Autodesk Fusion 360 part; units mm, degrees
sketch "Dimension" plane through (0, 0, 0) normal (0, 1, 0) x (1, 0, 0)
  line L0 (50, -40) -> (-50, -40)
  line L1 (-50, -40) -> (-50, 40)
  line L2 (-50, 40) -> (50, 40)
  line L3 (50, 40) -> (50, -40)
  line L4 (50, -40) -> (-50, 40) construction
  line L5 (-50, -40) -> (50, 40) construction
  dimension "d4" = 100
  dimension "d5" = 80
extrude "Extrude1" add sketch "Dimension" along normal blind 3
sketch "Stepper Mount" plane through (0, 3, 0) normal (0, 1, 0) x (-1, 0, 0)
  line L0 (-50, -40) -> (50, -40)
  line L1 (50, -40) -> (50, 40)
  line L2 (50, 40) -> (-50, 40)
  line L3 (-50, 40) -> (-50, -40)
  line L4 (30, -40) -> (-30, -40)
  line L5 (-30, -40) -> (-30, 40) construction
  line L6 (-30, 40) -> (30, 40)
  line L7 (30, 40) -> (30, -40) construction
  circle A0 centre (23.55, -33.85) radius 2.55
  circle A1 centre (-23.55, -33.85) radius 2.55
  circle A2 centre (23.55, 13.25) radius 2.55
  circle A3 centre (-23.55, 13.25) radius 2.55
  line L8 (-23.55, 13.25) -> (23.55, -33.85)
  circle A4 centre (15.49, -25.79) radius 2
  line L9 (0, -10.3) -> (-30, -10.3) construction
  line L10 (0, -10.3) -> (0, -40) construction
  circle A5 centre (-15.49, -25.79) radius 2
  line L11 (15.49, -25.79) -> (-15.49, 5.19)
  line L12 (-15.49, 5.19) -> (-16.9042, 3.7758) construction
  line L13 (-16.9042, 3.7758) -> (14.0758, -27.2042)
  line L14 (14.0758, -27.2042) -> (15.49, -25.79)
  line L15 (15.49, -25.79) -> (-15.49, 5.19)
  line L16 (-15.49, 5.19) -> (-14.0758, 6.6042) construction
  line L17 (-14.0758, 6.6042) -> (16.9042, -24.3758)
  line L18 (16.9042, -24.3758) -> (15.49, -25.79)
  line L19 (14.0758, 6.6042) -> (-16.9042, -24.3758)
  line L20 (16.9042, 3.7758) -> (-14.0758, -27.2042)
  line L21 (23.55, 13.25) -> (13.5057, 3.2057) construction
  line L22 (1.4142, -8.8858) -> (-23.55, -33.85) construction
  arc A6 (16.9042, 3.7758) -> (14.0758, 6.6042) centre (15.49, 5.19) ccw
  arc A7 (-14.0758, 6.6042) -> (-16.9042, 3.7758) centre (-15.49, 5.19) ccw
  arc A8 (-13.5057, 3.2057) -> (-12.0173, 4.5457) centre (0, -10.3) ccw
  dimension "d8" = 60
  dimension "d9" = 38.2
  dimension "d10" = 30
  dimension "d11" = 29.7
  dimension "d12" = 5.1
  dimension "d13" = 6.45
  dimension "d14" = 6.15
  dimension "d15" = 5.1
  dimension "d16" = 6.15
  dimension "d17" = 53.55
  dimension "d18" = 5.1
  dimension "d19" = 6.45
  dimension "d20" = 53.25
  dimension "d21" = 5.1
  dimension "d22" = 53.25
  dimension "d23" = 53.55
  dimension "d24" = 14.51
  dimension "d25" = 14.21
  dimension "d26" = 4
  dimension "d27" = 2
  dimension "d28" = 2
extrude "Extrude2" cut sketch "Stepper Mount" against normal through all contours A0 | A3 | L8 A4 L14 | L8 A4 L18 | L8 A4 L11 L14 L15 | L8 A4 L11 L15 L18 | L8 A4 L11 L13 L15 A8 | L8 A4 L11 L15 L17 A8 | L13 L20 A8 | L8 L11 L13 L15 L20 A8 | L8 L11 L15 L17 L20 A8 | L17 L20 A8 | L13 L19 L20 A8 | L8 L11 L13 L15 L19 L20 | A5 L19 L20 A8 | L8 L11 L15 L17 L19 L20 | L17 L19 L20 A8 | L19 L20 A6 A8 | L13 L19 A8 | L8 L11 L13 L15 L19 A8 | A5 | L8 L11 L15 L17 L19 A7 | L17 L19 A8 | L8 L11 L13 L15 A7 A8 | A1 | A2
sketch "Idler Mount" plane through (0, 3, 0) normal (0, 1, 0) x (-1, 0, 0)
  circle A0 centre (23.55, 13.25) radius 2.55
  circle A1 centre (23.55, -33.85) radius 2.55
  line L0 (14.8457, -22.3173) -> (16.9042, -24.3758)
  arc A2 (14.0758, -27.2042) -> (16.9042, -24.3758) centre (15.49, -25.79) ccw
  line L1 (14.0758, -27.2042) -> (12.0173, -25.1457)
  arc A3 (-12.0173, -25.1457) -> (12.0173, -25.1457) centre (0, -10.3) ccw
  line L2 (-12.0173, -25.1457) -> (-14.0758, -27.2042)
  arc A4 (-16.9042, -24.3758) -> (-14.0758, -27.2042) centre (-15.49, -25.79) ccw
  line L3 (-16.9042, -24.3758) -> (-14.8457, -22.3173)
  arc A5 (-14.8457, 1.7173) -> (-14.8457, -22.3173) centre (0, -10.3) ccw
  line L4 (-14.8457, 1.7173) -> (-16.9042, 3.7758)
  arc A6 (-14.0758, 6.6042) -> (-16.9042, 3.7758) centre (-15.49, 5.19) ccw
  line L5 (-14.0758, 6.6042) -> (-12.0173, 4.5457)
  arc A7 (12.0173, 4.5457) -> (-12.0173, 4.5457) centre (0, -10.3) ccw
  line L6 (12.0173, 4.5457) -> (14.0758, 6.6042)
  arc A8 (16.9042, 3.7758) -> (14.0758, 6.6042) centre (15.49, 5.19) ccw
  line L7 (16.9042, 3.7758) -> (14.8457, 1.7173)
  arc A9 (14.8457, -22.3173) -> (14.8457, 1.7173) centre (0, -10.3) ccw
  circle A10 centre (-23.55, 13.25) radius 2.55
  circle A11 centre (-23.55, -33.85) radius 2.55
  line L8 (-50, -40) -> (50, -40)
  line L9 (50, -40) -> (50, 40)
  line L10 (50, 40) -> (-50, 40)
  line L11 (-50, 40) -> (-50, -40)
  arc A12 (-14.8457, 1.7173) -> (-14.8457, -22.3173) centre (0, -10.3) ccw
  arc A13 (-12.0173, -25.1457) -> (12.0173, -25.1457) centre (0, -10.3) ccw
  arc A14 (14.8457, -22.3173) -> (14.8457, 1.7173) centre (0, -10.3) ccw
  arc A15 (12.0173, 4.5457) -> (-12.0173, 4.5457) centre (0, -10.3) ccw
  circle A16 centre (0, -10.3) radius 6 construction
  line L12 (0, -10.3) -> (50, -10.3) construction
  line L13 (0, -10.3) -> (-50, -10.3) construction
  circle A17 centre (0, -10.3) radius 9
  line L14 (6, -10.3) -> (-6, -10.3)
  line L15 (-6, -10.3) -> (-6, 40) construction
  line L16 (-6, 40) -> (6, 40)
  line L17 (6, 40) -> (6, -10.3) construction
  line L18 (50, 30) -> (-50, 30) construction
  line L19 (-50, 30) -> (-50, 40)
  line L20 (-50, 40) -> (50, 40)
  line L21 (50, 40) -> (50, 30)
  circle A18 centre (12, 30) radius 6 construction
  circle A19 centre (12, 30) radius 9 construction
  circle A20 centre (12, 30) radius 3
  line L22 (0, 20) -> (0, 2.5)
  circle A21 centre (-12, 30) radius 9 construction
  circle A22 centre (-12, 30) radius 6 construction
  circle A23 centre (-12, 30) radius 3
  dimension "d30" = 12
  dimension "d31" = 18
  dimension "d33" = 10
  dimension "d38" = 12
  dimension "d39" = 18
  dimension "d41" = 6
extrude "Extrude3" cut sketch "Idler Mount" against normal through all contours A20 | A23
sketch "Bracket Mount" plane through (0, 3, 0) normal (0, 1, 0) x (-1, 0, 0)
  circle A0 centre (12, 30) radius 3
  circle A1 centre (-12, 30) radius 3
  circle A2 centre (23.55, 13.25) radius 2.55
  circle A3 centre (23.55, -33.85) radius 2.55
  line L0 (14.8457, -22.3173) -> (16.9042, -24.3758)
  arc A4 (14.0758, -27.2042) -> (16.9042, -24.3758) centre (15.49, -25.79) ccw
  line L1 (14.0758, -27.2042) -> (12.0173, -25.1457)
  arc A5 (-12.0173, -25.1457) -> (12.0173, -25.1457) centre (0, -10.3) ccw
  line L2 (-12.0173, -25.1457) -> (-14.0758, -27.2042)
  arc A6 (-16.9042, -24.3758) -> (-14.0758, -27.2042) centre (-15.49, -25.79) ccw
  line L3 (-16.9042, -24.3758) -> (-14.8457, -22.3173)
  arc A7 (-14.8457, 1.7173) -> (-14.8457, -22.3173) centre (0, -10.3) ccw
  line L4 (-14.8457, 1.7173) -> (-16.9042, 3.7758)
  arc A8 (-14.0758, 6.6042) -> (-16.9042, 3.7758) centre (-15.49, 5.19) ccw
  line L5 (-14.0758, 6.6042) -> (-12.0173, 4.5457)
  arc A9 (12.0173, 4.5457) -> (-12.0173, 4.5457) centre (0, -10.3) ccw
  line L6 (12.0173, 4.5457) -> (14.0758, 6.6042)
  arc A10 (16.9042, 3.7758) -> (14.0758, 6.6042) centre (15.49, 5.19) ccw
  line L7 (16.9042, 3.7758) -> (14.8457, 1.7173)
  arc A11 (14.8457, -22.3173) -> (14.8457, 1.7173) centre (0, -10.3) ccw
  circle A12 centre (-23.55, 13.25) radius 2.55
  circle A13 centre (-23.55, -33.85) radius 2.55
  line L8 (-50, -40) -> (50, -40)
  line L9 (50, -40) -> (50, 40)
  line L10 (50, 40) -> (-50, 40)
  line L11 (-50, 40) -> (-50, -40)
  circle A14 centre (44, -32) radius 3.05
  line L12 (0, 20) -> (0, 2.5)
  circle A15 centre (-44, -32) radius 3.05
  line L13 (-2.5, 0) -> (-20, 0)
  circle A16 centre (44, 32) radius 3.05
  circle A17 centre (-44, 32) radius 3.05
  line L14 (-44, 32) -> (-44, -32) construction
  line L15 (44, -32) -> (44, 32) construction
  circle A18 centre (44, 0) radius 3.05
  circle A19 centre (-44, 0) radius 3.05
  dimension "d45" = 6.1
  dimension "d46" = 8
  dimension "d47" = 6
  dimension "d53" = 6.1
extrude "Extrude4" cut sketch "Bracket Mount" against normal through all contours A14 | A15 | A16 | A17 | A18 | A19
fillet "Fillet1" radius 5 4 edges at (50, 1.5, -40) (-50, 1.5, -40) (-50, 1.5, 40) (50, 1.5, 40)
equation "PlateWidth = 100 mm"
equation "PlateHeight = 80 mm"
equation "PlateThickness = 3 mm"
equation "d4 = PlateWidth"
equation "d5 = PlateHeight"
equation "d6 = PlateThickness"
equation "IdlerToBaseDistance = 10 mm"
equation "d33 = IdlerToBaseDistance"
equation "IdlerInternalDiameter = 12 mm"
equation "IdlerOuterDiameter = 18 mm"
equation "DriverInnerDiameter = 12 mm"
equation "DriverOuterDiameter = 18 mm"
equation "d38 = IdlerInternalDiameter"
equation "d39 = IdlerOuterDiameter"
equation "IdlerBoreDiameter = 6 mm"
equation "d41 = IdlerBoreDiameter"
equation "BracketMountHoleDiameter = 6.1 mm"
equation "BracketMountHoleHDistance = 6 mm"
equation "d45 = BracketMountHoleDiameter"
equation "d46 = BracketMountHoleVDistance"
equation "d47 = BracketMountHoleHDistance"
equation "BracketFilletRadius = 5 mm"
equation "d51 = BracketFilletRadius"
equation "BracketMountHoleVDistance = 8 mm"
equation "d53 = BracketMountHoleDiameter"
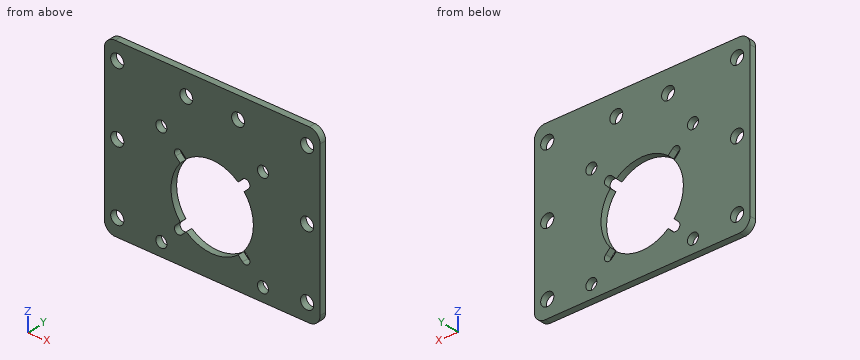
Check sheet for the modelled part. Datum: model origin and axes. Units: mm. Give positions to 0.01 mm unless a question says otherwise; leave off trailing zeros. Write each loop counter-clockwise with the first axis right and the second up, starting at its lowest first coordinate (ties: lowest second). Pieces come first, ordered by that corner, then holes. Notation, with made-up numbers: (85, 89.25) -> (99, 89.25) arc R13 cw to (99, 110.25) -> close; hole circle Ø11 at (10, 76). An arc over 180 degrees is marked (long way). Use one line per item in the form item = value. Start each with the question number.
1. Section check B-B (z = -33.85). Record the cut outline in (x, y), and give its area (3 significant figures).
2. Section check D-D (z = -10.5). Record the cut outline in (x, y), and give its area (3 significant figures).
3. Section check A-A (x = 23.55). Record the cut outline in (y, z), and give its area (3 significant figures).
4. Section check C-C (z = 0). Record the cut outline in (x, y).
5. Thickness scan on line 1 along Z through (x, y) = (44, 2.35); line 2 along Z through (x, y) = (23.55, 1.85); line 3 along Z through (x, y) = (16, 1.8). Record the ranges inside material, lowest first. Write a range as from..to.
Conclusion:
q1.outline = (-50, 0) -> (-46.42, 0) -> (-46.42, 3) -> (-50, 3) -> close; (-41.58, 0) -> (-26.1, 0) -> (-26.1, 3) -> (-41.58, 3) -> close; (-21, 0) -> (21, 0) -> (21, 3) -> (-21, 3) -> close; (26.1, 0) -> (41.58, 0) -> (41.58, 3) -> (26.1, 3) -> close; (46.42, 0) -> (50, 0) -> (50, 3) -> (46.42, 3) -> close
q1.area = 240 mm²
q2.outline = (-50, 0) -> (-19.1, 0) -> (-19.1, 3) -> (-50, 3) -> close; (19.1, 0) -> (50, 0) -> (50, 3) -> (19.1, 3) -> close
q2.area = 185 mm²
q3.outline = (0, -40) -> (3, -40) -> (3, -36.4) -> (0, -36.4) -> close; (0, -31.3) -> (3, -31.3) -> (3, 10.7) -> (0, 10.7) -> close; (0, 15.8) -> (3, 15.8) -> (3, 40) -> (0, 40) -> close
q3.area = 209 mm²
q4.outline = (-50, 0) -> (-47.05, 0) -> (-47.05, 3) -> (-50, 3) -> close; (-40.95, 0) -> (-16.09, 0) -> (-16.09, 3) -> (-40.95, 3) -> close; (16.08, 0) -> (40.95, 0) -> (40.95, 3) -> (16.08, 3) -> close; (47.05, 0) -> (50, 0) -> (50, 3) -> (47.05, 3) -> close
q5.line_1 = -40..-35.05, -28.95..-3.05, 3.05..28.95, 35.05..40
q5.line_2 = -40..-36.4, -31.3..10.7, 15.8..40
q5.line_3 = -40..-27.72, -23.47..-20.73, 0.13..2.87, 7.12..40
